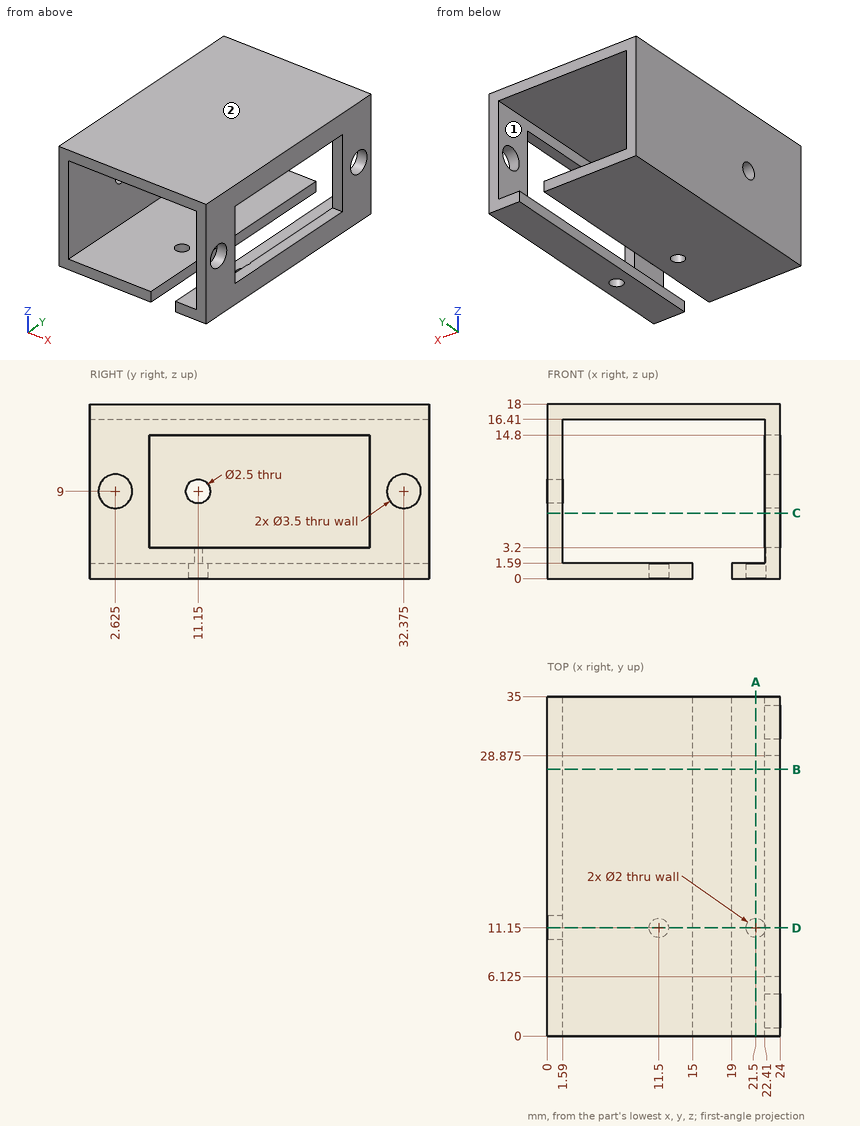
Source: three-view drawing plus pictorial views. Frame: mm from the lowest corner of the part. A direction names the side the tool comes from. Coordinates: 2 decimals unless noted, no trailing zeros. Loops run counter-clockwise (first coordinate to the right, second up) from the corner with the lowest first, then second, coordinate; pieces in that order, holes last. Notation, with made-up numbers: (-34.5, -6) - (16.5, -6) arc R32 cw to (16.5, 33) - close; hole circle Ø1 at (-4, -20.75). An arc over 180 degrees is marked (long way). One line per item, written item: value. Start each with the question number.
1. Section A-A (x = 21.5). Return the cut outline in (y, z), and give its area (3 significant figures).
2. Ray query, L1, parallel to Z at x = 22, y = 23; L2, parallel to X at y = 4, z = 11.75; L3, parallel to Y at x = 11.5, z = 0.9. Return the intervals inside material, ascending.
3. Section D-D (y = 11.15). Return the cut outline in (x, z), and give its area (3 significant figures).
4. Section C-C (z = 6.75). Return the cut outline in (x, y) (3 decimals), and give its area (3 significant figures).
5. Set-up query: the marked faces 1 and 2. Return all of +Z, -Z, +X, -X, +Y, -Y with unobstructed straight access to the full face (end or side cutting, diameter ignored); none if empty.
6. Contact query for flat-ended pins moving along their axis: P1, Ø1, axis at x = 2.5, y = 13.5, coming from the -Z side; P2, Ø2, axis at y = 32.375, z = 9, coming from the +X side. Output: stop coordinate, or through.
7. Section B-B (y = 27.5). Return the cut outline in (x, z), and give its area (3 significant figures).
Verdict:
1. outline: (0, 0) - (10.15, 0) - (10.15, 1.59) - (0, 1.59) - close; (0, 16.41) - (35, 16.41) - (35, 18) - (0, 18) - close; (12.15, 0) - (35, 0) - (35, 1.59) - (12.15, 1.59) - close
1. area: 108 mm2
2. L1: z = 0 to 1.59, 16.41 to 18
2. L2: x = 0 to 1.59, 22.41 to 24
2. L3: y = 0 to 10.15, 12.15 to 35
3. outline: (0, 0) - (10.5, 0) - (10.5, 1.59) - (1.59, 1.59) - (1.59, 7.75) - (0, 7.75) - close; (0, 10.25) - (1.59, 10.25) - (1.59, 16.41) - (22.41, 16.41) - (22.41, 14.8) - (24, 14.8) - (24, 18) - (0, 18) - close; (12.5, 0) - (15, 0) - (15, 1.59) - (12.5, 1.59) - close; (19, 0) - (20.5, 0) - (20.5, 1.59) - (19, 1.59) - close; (22.5, 0) - (24, 0) - (24, 3.2) - (22.5, 3.2) - close
3. area: 88.2 mm2
4. outline: (0, 0) - (1.59, 0) - (1.59, 35) - (0, 35) - close; (22.41, 0) - (24, 0) - (24, 6.125) - (22.41, 6.125) - close; (22.41, 28.875) - (24, 28.875) - (24, 35) - (22.41, 35) - close
4. area: 75.1 mm2
5. face 1: +Y, -Y
5. face 2: +Z, +X, -X, +Y, -Y
6. P1: stops at z = 0
6. P2: stops at x = 1.59
7. outline: (0, 0) - (15, 0) - (15, 1.59) - (1.59, 1.59) - (1.59, 16.41) - (22.41, 16.41) - (22.41, 14.8) - (24, 14.8) - (24, 18) - (0, 18) - close; (19, 0) - (24, 0) - (24, 3.2) - (22.41, 3.2) - (22.41, 1.59) - (19, 1.59) - close
7. area: 98.6 mm2
